from build123d import *

# Parameters (mm, degrees)
CUT_EXTRUDE1_DEPTH = 0.79375
FILLET2_R          = 0.79375
FILLET3_R          = 0.396875
CHAMFER1_SIZE      = 0.254
CHAMFER2_SIZE      = 0.127


with BuildPart() as part:
    # Sketch1 → Revolve1 (revolve)
    with BuildSketch(Plane.XY):
        Polygon((0, 0), (2.38125, 0), (2.38125, 19.05), (4.7625, 19.05), (4.7625, 20.6375), (0, 20.6375), align=None)
    revolve(axis=Axis((0, 5.173549107, 0), (0, -1, 0)))

    # Sketch2 → Cut-Extrude1 (cut)
    with BuildSketch(Plane(origin=(0, 20.6375, 0), x_dir=(1, 0, 0), z_dir=(0, 1, 0))):
        Polygon((-3.175, 0.79375), (-0.79375, 0.79375), (-0.79375, 3.175), (0.79375, 3.175), (0.79375, 0.79375), (3.175, 0.79375), (3.175, -0.79375), (0.79375, -0.79375), (0.79375, -3.175), (-0.79375, -3.175), (-0.79375, -0.79375), (-3.175, -0.79375), align=None)
    extrude(amount=-CUT_EXTRUDE1_DEPTH, mode=Mode.SUBTRACT)

    # Fillet2
    fillet2_edges = [part.edges().sort_by_distance(p)[0] for p in [
        (-4.7625, 20.6375, 0),
        (-2.38125, 19.05, 0),
    ]]
    fillet(fillet2_edges, radius=FILLET2_R)

    # Fillet3
    fillet3_edges = [part.edges().sort_by_distance(p)[0] for p in [
        (-3.175, 20.240625, -0.79375),
        (-0.79375, 20.240625, -0.79375),
        (-0.79375, 20.240625, -3.175),
        (0.79375, 20.240625, -3.175),
        (0.79375, 20.240625, -0.79375),
        (3.175, 20.240625, -0.79375),
        (3.175, 20.240625, 0.79375),
        (0.79375, 20.240625, 0.79375),
        (0.79375, 20.240625, 3.175),
        (-0.79375, 20.240625, 3.175),
        (-0.79375, 20.240625, 0.79375),
        (-3.175, 20.240625, 0.79375),
        (-1.984375, 19.84375, -0.79375),
        (-0.79375, 19.84375, -1.984375),
        (0, 19.84375, -3.175),
        (0.79375, 19.84375, -1.984375),
        (1.984375, 19.84375, -0.79375),
        (3.175, 19.84375, 0),
        (1.984375, 19.84375, 0.79375),
        (0.79375, 19.84375, 1.984375),
        (0, 19.84375, 3.175),
        (-0.79375, 19.84375, 1.984375),
        (-1.984375, 19.84375, 0.79375),
        (-3.175, 19.84375, 0),
    ]]
    fillet(fillet3_edges, radius=FILLET3_R)

    # Chamfer1
    chamfer1_edges = [part.edges().sort_by_distance(p)[0] for p in [
        (-4.7625, 19.05, 0),
        (-2.38125, 0, 0),
    ]]
    chamfer(chamfer1_edges, length=CHAMFER1_SIZE)

    # Chamfer2
    chamfer2_edges = [part.edges().sort_by_distance(p)[0] for p in [
        (-1.984375, 20.6375, -0.79375),
        (-0.79375, 20.6375, -1.984375),
        (0, 20.6375, -3.175),
        (0.79375, 20.6375, -1.984375),
        (1.984375, 20.6375, -0.79375),
        (3.175, 20.6375, 0),
        (1.984375, 20.6375, 0.79375),
        (0.79375, 20.6375, 1.984375),
        (0, 20.6375, 3.175),
        (-0.79375, 20.6375, 1.984375),
        (-1.984375, 20.6375, 0.79375),
        (-3.175, 20.6375, 0),
        (-0.909991996, 20.6375, -0.909991996),
        (0.909991996, 20.6375, -0.909991996),
        (0.909991996, 20.6375, 0.909991996),
        (-0.909991996, 20.6375, 0.909991996),
        (-3.058758004, 20.6375, -0.677508004),
        (-3.058758004, 20.6375, 0.677508004),
        (-0.677508004, 20.6375, 3.058758004),
        (0.677508004, 20.6375, 3.058758004),
        (3.058758004, 20.6375, 0.677508004),
        (3.058758004, 20.6375, -0.677508004),
        (-0.677508004, 20.6375, -3.058758004),
        (0.677508004, 20.6375, -3.058758004),
    ]]
    chamfer(chamfer2_edges, length=CHAMFER2_SIZE)


solid = part.part
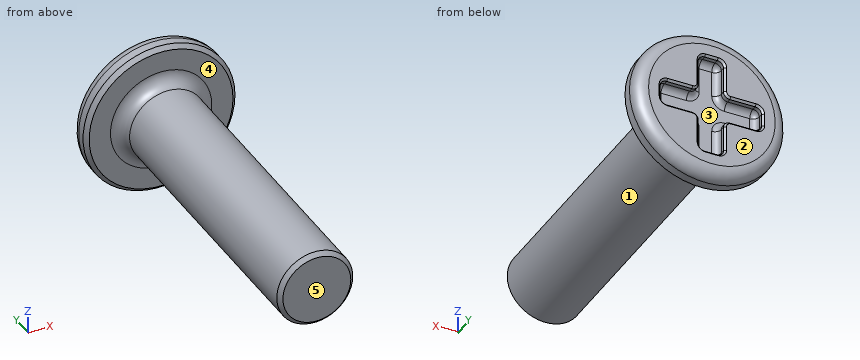
For this review, take the finished solid that the model builds, in its own axes (mm). Face numbers are marked on the shaded views. A direction names the side the tool comes from. Give positions to 0.01 mm unless a question says otherwise; leave off trailing zeros. Order: outer loops, then holes, each group sorted by start corner. A loop starts at its lowest first (then second) coordinate and runs counter-clockwise, first axis right, second up. Notation, with made-up numbers: (77, 82.25) -> (90, 82.25) arc R25 ccw to (90, 121.25) -> close; hole circle Ø7 at (9, -31). An arc over 180 degrees is marked (long way). Write item = value, one per line.
1) Draft analysis for pull direction Z (two halves, no side actions). For the marked faces 1, 2 and 3, state which applies: pulls with the +Z half, pulls with the -Z half, needs draft (parallel to the pull), parting line crosses it, or undercut.
Findings:
face_1 = parting line crosses it
face_2 = needs draft
face_3 = undercut
2) Insertion check: pin 1 (3 mm diameter, centred on x = 1, y = 12.5, fed in from -Z); pin 2 (1 mm diameter, centred on y = 4.5, z = 0, fed in from -X). Each pin has a flat end and moves straight along its axis. Give the tip position at first contact, or say it passes through.
Findings:
pin_1 = -2.38
pin_2 = -2.38
3) For the marked faces 4 and 5, list the 3-axis set-ups (+Z, -Z, +X, -X, +Y, -Y) from which the entire face can be reached by the end or side of a thin tool; tool diameter is ignored.
Findings:
face_4 = -Y
face_5 = +Z, -Z, +X, -X, -Y
4) To check wall thickness, follow L1, parallel to Y at x = -1.25, z = -3.25; L2, parallel to Y at x = 0.5, z = -0.75; L3, parallel to X at y = 12, z = 1.5. State the ranges of each line that lie inside material, in increasing order. Write a range as from..to.
Findings:
L1 = 19.05..20.64
L2 = 0..19.84
L3 = -1.85..1.85
5) We need section C-C, the plane y = 10.5. Give the boundary of the cut face in (x, z).
Findings:
outline = circle Ø4.76 at (0, 0)
